from build123d import *

# Parameters (mm, degrees)
SKETCH_W            = 120
SKETCH_H            = 100
PAD_DEPTH           = 10
SKETCH001_W         = 120
SKETCH001_H         = 30
PAD001_DEPTH        = 10
POCKET_DEPTH        = 36
SKETCH003_W         = 80
SKETCH003_H         = 6
PAD002_DEPTH        = 30
SKETCH004_R         = 2.75
HOLE_DEPTH          = 10.001
SKETCH005_W         = 7
SKETCH005_H         = 25
PAD003_DEPTH        = 25
SKETCH006_R         = 5.5
HOLE001_DEPTH       = 130.001
SKETCH011_R         = 7.5
HOLE004_DEPTH       = 25
HOLE004_TIPS_R      = 7.5
HOLE005_D           = 5.5
HOLE005_DEPTH       = 25
HOLE005_CBORE_D     = 13
HOLE005_CBORE_DEPTH = 6.4
SKETCH013_R         = 7.5
HOLE006_DEPTH       = 170.001
SKETCH014_R         = 7.5
HOLE007_DEPTH       = 25


with BuildPart() as part:
    # Sketch → Pad (new body)
    with BuildSketch(Plane.XY):
        with Locations((0, -120)):
            Rectangle(SKETCH_W, SKETCH_H)
    extrude(amount=PAD_DEPTH)

    # Sketch001 → Pad001 (join)
    with BuildSketch(Plane.XZ.offset(70)):
        with Locations((0, -15)):
            Rectangle(SKETCH001_W, SKETCH001_H)
    extrude(amount=PAD001_DEPTH)

    # Sketch002 → Pocket (cut)
    with BuildSketch(Plane.XY):
        Polygon((-60, -170), (-60, -90), (-40, -170), align=None)
        Polygon((60, -170), (60, -90), (40, -170), align=None)
    extrude(amount=POCKET_DEPTH, mode=Mode.SUBTRACT)

    # Sketch003 → Pad002 (join)
    with BuildSketch(Plane.XY):
        with Locations((0, -167)):
            Rectangle(SKETCH003_W, SKETCH003_H)
    extrude(amount=-PAD002_DEPTH)

    # Sketch004 → Hole (cut, through all)
    with BuildSketch(Plane.XZ.offset(160)):
        with Locations((-30, -15)):
            Circle(SKETCH004_R)
        with Locations((30, -15)):
            Circle(SKETCH004_R)
    extrude(amount=HOLE_DEPTH, mode=Mode.SUBTRACT)

    # Sketch005 → Pad003 (join)
    with BuildSketch(Plane.XY):
        with Locations((43.5, -127.5)):
            Rectangle(SKETCH005_W, SKETCH005_H)
        with Locations((-43.5, -127.5)):
            Rectangle(SKETCH005_W, SKETCH005_H)
    extrude(amount=-PAD003_DEPTH)

    # Sketch006 → Hole001 (cut, through all)
    with BuildSketch(Plane.YZ.offset(70)):
        with Locations((-127.5, -12.5)):
            Circle(SKETCH006_R)
    extrude(amount=-HOLE001_DEPTH, mode=Mode.SUBTRACT)

    # Sketch011 → Hole004 (cut)
    with BuildSketch(Plane.XZ.offset(170)):
        with Locations((0, -15)):
            Circle(SKETCH011_R)
    extrude(amount=-HOLE004_DEPTH, mode=Mode.SUBTRACT)

    # Hole004 tips → Hole004 tip 1 section 0
    with BuildSketch(Plane.XZ.offset(145), mode=Mode.PRIVATE) as hole004_tip_1_s0:
        with Locations((0, -15)):
            Circle(HOLE004_TIPS_R)
    loft([hole004_tip_1_s0.sketch, Vertex(0, -140.493545, -15)], mode=Mode.SUBTRACT)

    # Hole005
    with Locations(Plane.XZ.offset(80)):
        with Locations((-30, -15), (30, -15)):
            CounterBoreHole(HOLE005_D / 2, HOLE005_CBORE_D / 2, HOLE005_CBORE_DEPTH, depth=HOLE005_DEPTH)

    # Sketch013 → Hole006 (cut, through all)
    with BuildSketch(Plane.XZ):
        with Locations((0, -15)):
            Circle(SKETCH013_R)
    extrude(amount=HOLE006_DEPTH, mode=Mode.SUBTRACT)

    # Sketch014 → Hole007 (cut)
    with BuildSketch(Plane.XY):
        with Locations((0, -130)):
            Circle(SKETCH014_R)
    extrude(amount=HOLE007_DEPTH, mode=Mode.SUBTRACT)


solid = part.part
Here's how the part is built. I have some questions about the finished solid (model axes, mm). A direction names the side the tool comes from. Round coordinates to 2 decimals unless told otherwise and drop trailing zeros. Write each loop counter-clockwise with the first axis right and the second up, starting at its lowest first coordinate (ties: lowest second). Pieces come first, ordered by that corner, then holes.
1. If we mould it in two halves opening along Y, with no side actions, what happens to faces 6 (the flat face through (-50.14, -129.44, 4.93)), 7 (the flat face through (43, -115, -12)), 8 (the flat face through (40, -167, -15))? For each: released by +Y, released by -Y, zero draft, split by the parting line, or undercut.
2. Suppose I cut it at B-B (x = 43.5). List the corners of the cut face in (y, z) for me, and give its area (3 significant figures).
3. Will these pins go through, and if not, where does the flat tip stop? pin 1 Ø4.5 at (x, z) = (-30, -15) entering from -Y; pin 2 Ø2 at (x, y) = (42, -129) entering from -Z; pin 3 Ø14.5 at (y, z) = (-127.5, -12.5) entering from -X; pin 4 Ø3.5 at (x, z) = (-42.5, -7) entering from -Y.
4. Suppose I cut it at C-C (z = -5.5). List the corners of the cut face in (x, y) for me, and give its area (3 significant figures).
5. I need wall thicknesses on L1, parallel to Y at x = 16.5, z = -15; L2, parallel to Z at x = 0, y = -74; L3, parallel to X at y = -117, z = -3. Which ranges of each line are inside material? Lowest first, please.
6. For faces 1 (the flat face through (-44, -140, -12)), 2 (the flat face through (-1, -80, -5)), 3 (the flat face through (50.14, -129.44, 4.93)), 4 (the flat face through (47, -127.7, -6.8)), 5 (the flat face through (-47, -127.7, -6.8)), which set-ups out of +Z, -Z, +X, -X, +Y, -Y let a thin tool reach every point of the face, with its end or its side?
7. Suppose I cut it at A-A (z = 7). List the corners of the cut face in (x, y) for me.
8. Suppose I cut it at D-D (x = -30). List the corners of the cut face in (y, z) for me.
Answer sheet:
1. face 6: released by -Y
1. face 7: undercut
1. face 8: zero draft
2. outline: (-156, 0) - (-140, 0) - (-140, -25) - (-115, -25) - (-115, 0) - (-80, 0) - (-80, -30) - (-70, -30) - (-70, 10) - (-156, 10) - close; hole circle Ø11 at (-127.5, -12.5)
2. area: 1,690 mm2
3. pin 1: passes through
3. pin 2: stops at z = -25
3. pin 3: stops at x = -47
3. pin 4: stops at y = -140
4. outline: (-60, -80) - (60, -80) - (60, -70) - (-60, -70) - close; (-47, -140) - (-40, -140) - (-40, -115) - (-47, -115) - close; (-40, -170) - (40, -170) - (40, -164) - (-40, -164) - close; (40, -140) - (47, -140) - (47, -115) - (40, -115) - close
4. area: 2,030 mm2
5. L1: y = -170 to -164, -80 to -70
5. L2: z = -30 to -22.5, -7.5 to 10
5. L3: x = -47 to -40, 40 to 47
6. face 1: -Z, +X, -X, -Y
6. face 2: -Z, +X, -X
6. face 3: +Z, -Z, +X, -Y
6. face 4: -Z, +X, -Y
6. face 5: -Z, -X, -Y
7. outline: (-60, -90) - (-40, -170) - (40, -170) - (60, -90) - (60, -70) - (-60, -70) - close; hole circle Ø15 at (0, -130)
8. outline: (-170, -30) - (-164, -30) - (-164, -17.75) - (-170, -17.75) - close; (-170, -12.25) - (-164, -12.25) - (-164, 0) - (-80, 0) - (-80, -8.5) - (-73.6, -8.5) - (-73.6, -12.25) - (-70, -12.25) - (-70, 10) - (-170, 10) - close; (-80, -30) - (-70, -30) - (-70, -17.75) - (-73.6, -17.75) - (-73.6, -21.5) - (-80, -21.5) - close
